Can you work these out from the model? Positions are in its coordinate system, mm. Face numbers are marked on the shaded views. A direction names the side the tool comes from. Coordinates: 2 decimals unless noted, no trailing zeros. Order: outer loops, then holes, each group sorted by start corner. A loop starts at its lowest first (then second) coordinate and runs counter-clockwise, first axis right, second up.
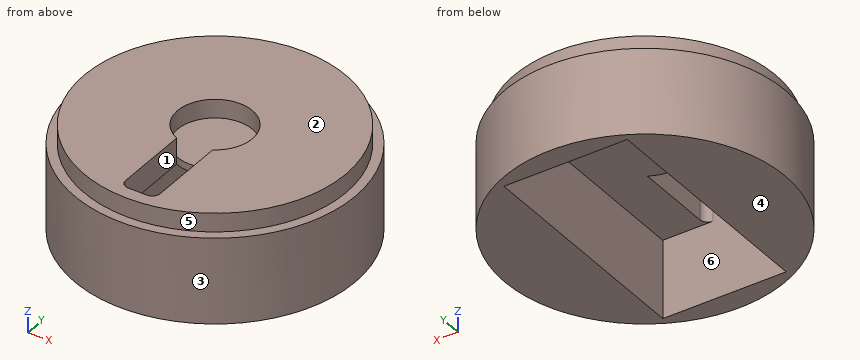
```python
from build123d import *

# Parameters (mm, degrees)
F0_R      = 37.5
F1_DEPTH  = 28
F2_W      = 33
F2_H      = 63
F3_DEPTH  = 21
F4_R      = 10
F5_DEPTH  = 5
F7_DEPTH  = 25
F9_DEPTH  = 15
F10_R     = 37.5
F10_R_2   = 35
F11_DEPTH = 5


with BuildPart() as f1:
    # F0 (on Top) → F1 (new body)
    with BuildSketch(Plane.XY):
        Circle(F0_R)
    extrude(amount=F1_DEPTH)

    # F2 (on face) → F3 (cut)
    with BuildSketch(Plane(origin=(0, 0, 0), x_dir=(1, 0, 0), z_dir=(0, 0, -1))):
        Rectangle(F2_W, F2_H)
    extrude(amount=-F3_DEPTH, mode=Mode.SUBTRACT)

    # F4 (on face) → F5 (cut)
    with BuildSketch(Plane.XY.offset(28)):
        Circle(F4_R)
    extrude(amount=-F5_DEPTH, mode=Mode.SUBTRACT)

    # F6 (on face) → F7 (cut)
    with BuildSketch(Plane(origin=(0, 0, 21), x_dir=(1, 0, 0), z_dir=(0, 0, -1))):
        with BuildLine():
            Line((3.0463133007, 31.5), (-1.9864209462, 31.5))
            ThreePointArc((-1.9864209462, 31.5), (-4.0973785389, 29.3890424073), (-1.9864209462, 27.2780848145))
            Line((-1.9864209462, 27.2780848145), (3.0463133007, 27.2780848145))
            ThreePointArc((3.0463133007, 27.2780848145), (5.1572708935, 29.3890424073), (3.0463133007, 31.5))
        make_face()
    extrude(amount=-F7_DEPTH, mode=Mode.SUBTRACT)

    # F8 (on face) → F9 (cut)
    with BuildSketch(Plane.XY.offset(28)):
        with BuildLine():
            Line((-4.0973785389, -9.1220331675), (-4.0973785389, -29.3890424073))
            ThreePointArc((-4.0973785389, -29.3890424073), (-3.4790933748, -27.8963699787), (-1.9864209462, -27.2780848145))
            Line((-1.9864209462, -27.2780848145), (3.0463133007, -27.2780848145))
            ThreePointArc((3.0463133007, -27.2780848145), (4.5389857293, -27.8963699787), (5.1572708935, -29.3890424073))
            Line((5.1572708935, -29.3890424073), (5.1572708935, -8.5675292198))
            ThreePointArc((5.1572708935, -8.5675292198), (0.5980899663, -9.9820983962), (-4.0973785389, -9.1220331675))
        make_face()
    extrude(amount=-F9_DEPTH, mode=Mode.SUBTRACT)

    # F10 (on face) → F11 (cut)
    with BuildSketch(Plane.XY.offset(28)):
        Circle(F10_R)
        Circle(F10_R_2, mode=Mode.SUBTRACT)
    extrude(amount=-F11_DEPTH, mode=Mode.SUBTRACT)


solid = f1.part
```
1. Imagine slicing it at D-D on x = -11. Please give me the cut outline in (y, z), then the cut area to 3 significant figures.
Completed:
outline: (-35.85, 0) - (-31.5, 0) - (-31.5, 21) - (31.5, 21) - (31.5, 0) - (35.85, 0) - (35.85, 23) - (33.23, 23) - (33.23, 28) - (-33.23, 28) - (-33.23, 23) - (-35.85, 23) - close
area: 658 mm2
2. Imagine slicing it at B-B on z = 8. Please give me the cut outline in (x, y), then the cut area to 3 significant figures.
Completed:
outline: circle Ø75 at (0, 0); hole (-16.5, -31.5) - (16.5, -31.5) - (16.5, 31.5) - (-16.5, 31.5) - close
area: 2,340 mm2
3. Imagine slicing it at C-C on y = 0. Please give me the cut outline in (x, z).
Completed:
outline: (-37.5, 0) - (-16.5, 0) - (-16.5, 21) - (16.5, 21) - (16.5, 0) - (37.5, 0) - (37.5, 23) - (35, 23) - (35, 28) - (10, 28) - (10, 23) - (-10, 23) - (-10, 28) - (-35, 28) - (-35, 23) - (-37.5, 23) - close
4. Please list where these lines run through material, in increasing order: probe 1 along Y at (x, z) = (13.5, 11.5); probe 2 along Y at (x, z) = (0, 26.1); probe 3 along Z at (x, y) = (-8, 9).
Completed:
probe 1: y = -34.99 to -31.5, 31.5 to 34.99
probe 2: y = -35 to -31.5, 10 to 35
probe 3: z = 21 to 28
5. On a 3-axis mill with a long thin cutter (end or side, diameter ignored), from which of +Z, -Z, +X, -X, +Y, -Y can I reach the whole of each face in a straight line? I mean the marked faces 4, 5 and 6. Say none if no direction works.
Completed:
face 4: -Z, +X, -X, +Y, -Y
face 5: +Z
face 6: -Z
6. Thinking about a two-plate mould opening in Y: for the marked faces 1, 2 and 3, which applies, pulls with the +Y half, pulls with the -Y half, needs draft (parallel to the pull), parting line crosses it, or undercut?
Completed:
face 1: undercut
face 2: needs draft
face 3: parting line crosses it
7. Imagine slicing it at A-A on x = 0. Please give me the cut outline in (y, z), then the cut area to 4 significant figures.
Completed:
outline: (-37.5, 0) - (-31.5, 0) - (-31.5, 28) - (-35, 28) - (-35, 23) - (-37.5, 23) - close; (-10, 21) - (31.5, 21) - (31.5, 0) - (37.5, 0) - (37.5, 23) - (35, 23) - (35, 28) - (10, 28) - (10, 23) - (-10, 23) - close
area: 501.5 mm2
8. I'm going to push flat-ended pins straight in: pin 1 (8.5 mm diameter, centred on x = 6, z = 10, fed in from +Y); pin 2 (10 mm diameter, centred on x = -19, y = 18.5, fed in from -Z); pin 3 (12 mm diameter, centred on y = -23.5, z = 15.5, fed in from -X); pin 4 (1.5 mm diameter, centred on y = 7, z = 11, fed in from -X). Where does each tip first touch, or does it pass through?
Completed:
pin 1: stops at y = 37.46
pin 2: stops at z = 0
pin 3: stops at x = -33.17
pin 4: stops at x = -36.98
